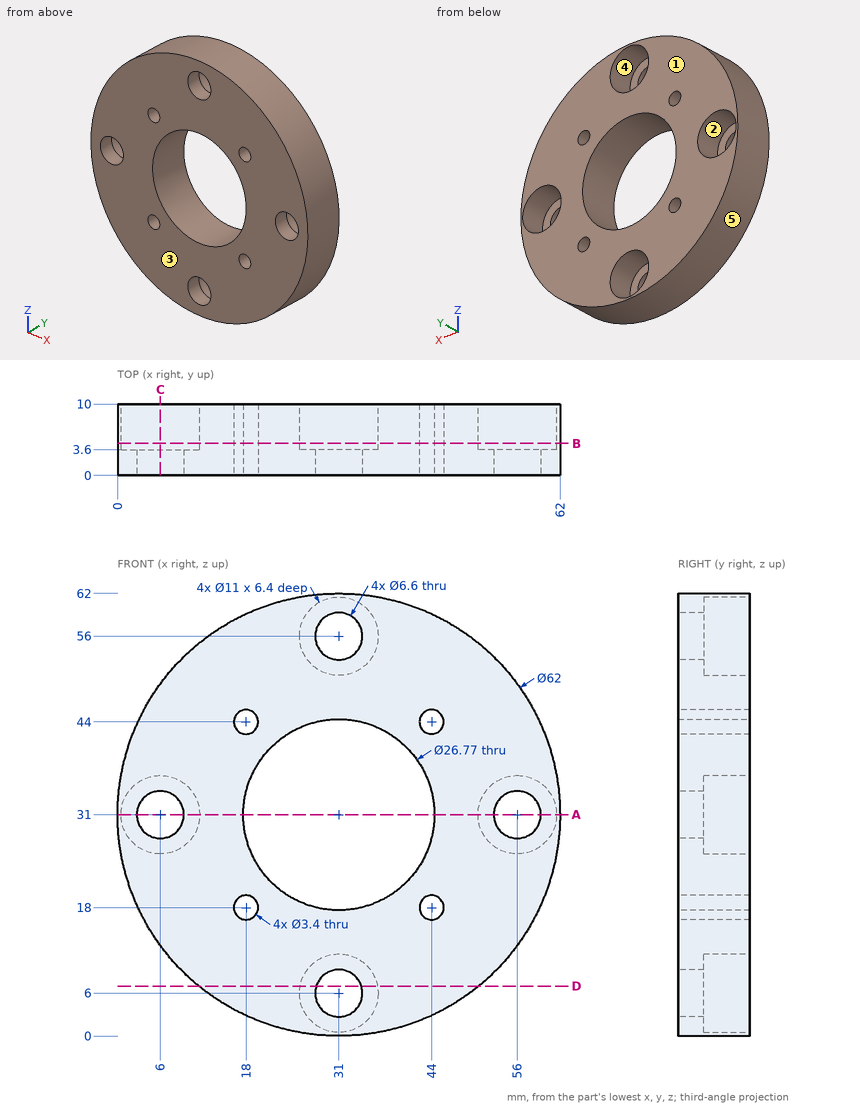
Job drawing, mm, ordinate dimensions from the low corner. One solid piece. A direction names the side the tool comes from. Round coordinates to 2 decimals unless told otherwise and drop trailing zeros. Loops run counter-clockwise (first coordinate to the right, second up) from the corner with the lowest first, then second, coordinate; pieces in that order, holes last. Notation, with made-up numbers: (-16, 76.5) -> (1, 76.5) arc R10 cw to (1, 84.5) -> close; hole circle Ø6 at (11.5, 75.5). An arc over 180 degrees is marked (long way). Use a Markdown table: item, result.
1) Cut at B-B, the plane y = 4.5. State how many separate pieces and enclosed holes the cut face has, and give its area (3 significant figures).
The answers:
| item | result |
|---|---|
| separate pieces | 1 |
| enclosed holes | 9 |
| area | 2,040 mm2 |
2) Probe line 1 (Z direction, x = 26, y = 8) (1 decimal); line 2 (X direction, y = 6, z = 34.5) (1 decimal); line 3 (X direction, y = 5, z = 16.5). List the from-to ranges inside material, lowest first. Write a range as [from, to].
The answers:
| item | result |
|---|---|
| line 1 | z = [0.4, 3.7], [8.3, 18.6], [43.4, 53.7], [58.3, 61.6] |
| line 2 | x = [0.2, 1.8], [10.2, 18.1], [43.9, 51.8], [60.2, 61.8] |
| line 3 | x = [3.6, 17.2], [18.8, 43.2], [44.8, 58.4] |
3) Pull direction Z, two halves, no side cores. Call the marked faces 3, 4 and 5: pulls with the +Z half, pulls with the -Z half, needs draft (parallel to the pull), parting line crosses it, or undercut.
The answers:
| item | result |
|---|---|
| face 3 | needs draft |
| face 4 | undercut |
| face 5 | parting line crosses it |
4) Tool access for the marked faces 1 and 2: list every direction of +Z, -Z, +X, -X, +Y, -Y with a clear straight run to the whole face (end or side of a thin tool).
The answers:
| item | result |
|---|---|
| face 1 | +Z, -Z, +X, -X, +Y |
| face 2 | +Y |
5) Cut at C-C, the plane x = 6. List the corners of the cut face in (y, z).
The answers:
| item | result |
|---|---|
| outline | (0, 12.67) -> (10, 12.67) -> (10, 25.5) -> (3.6, 25.5) -> (3.6, 27.7) -> (0, 27.7) -> close; (0, 34.3) -> (3.6, 34.3) -> (3.6, 36.5) -> (10, 36.5) -> (10, 49.33) -> (0, 49.33) -> close |
6) Cut at A-A, the plane z = 31. List the corners of the cut face in (x, y) (1 decimal), and give its area (3 significant figures).
The answers:
| item | result |
|---|---|
| outline | (0, 0) -> (2.7, 0) -> (2.7, 3.6) -> (0.5, 3.6) -> (0.5, 10) -> (0, 10) -> close; (9.3, 0) -> (17.6, 0) -> (17.6, 10) -> (11.5, 10) -> (11.5, 3.6) -> (9.3, 3.6) -> close; (44.4, 0) -> (52.7, 0) -> (52.7, 3.6) -> (50.5, 3.6) -> (50.5, 10) -> (44.4, 10) -> close; (59.3, 0) -> (62, 0) -> (62, 10) -> (61.5, 10) -> (61.5, 3.6) -> (59.3, 3.6) -> close |
| area | 164 mm2 |
7) Cut at D-D, the plane z = 7. List the corners of the cut face in (x, y) (1 decimal).
The answers:
| item | result |
|---|---|
| outline | (11.4, 0) -> (27.9, 0) -> (27.9, 3.6) -> (25.6, 3.6) -> (25.6, 10) -> (11.4, 10) -> close; (34.1, 0) -> (50.6, 0) -> (50.6, 10) -> (36.4, 10) -> (36.4, 3.6) -> (34.1, 3.6) -> close |
8) Drop flat-ended pins along their axis: pin 1 Ø6 at (x, y) = (35, 3) entering from +Z; pin 2 Ø3 at (x, z) = (27.5, 6.5) entering from +Y; pin 3 Ø4 at (x, y) = (20, 7.5) entering from +Z (1 decimal). Give the stop position or say it passes through.
The answers:
| item | result |
|---|---|
| pin 1 | stops at z = 61.98 |
| pin 2 | stops at y = 3.6 |
| pin 3 | stops at z = 60.7 |
